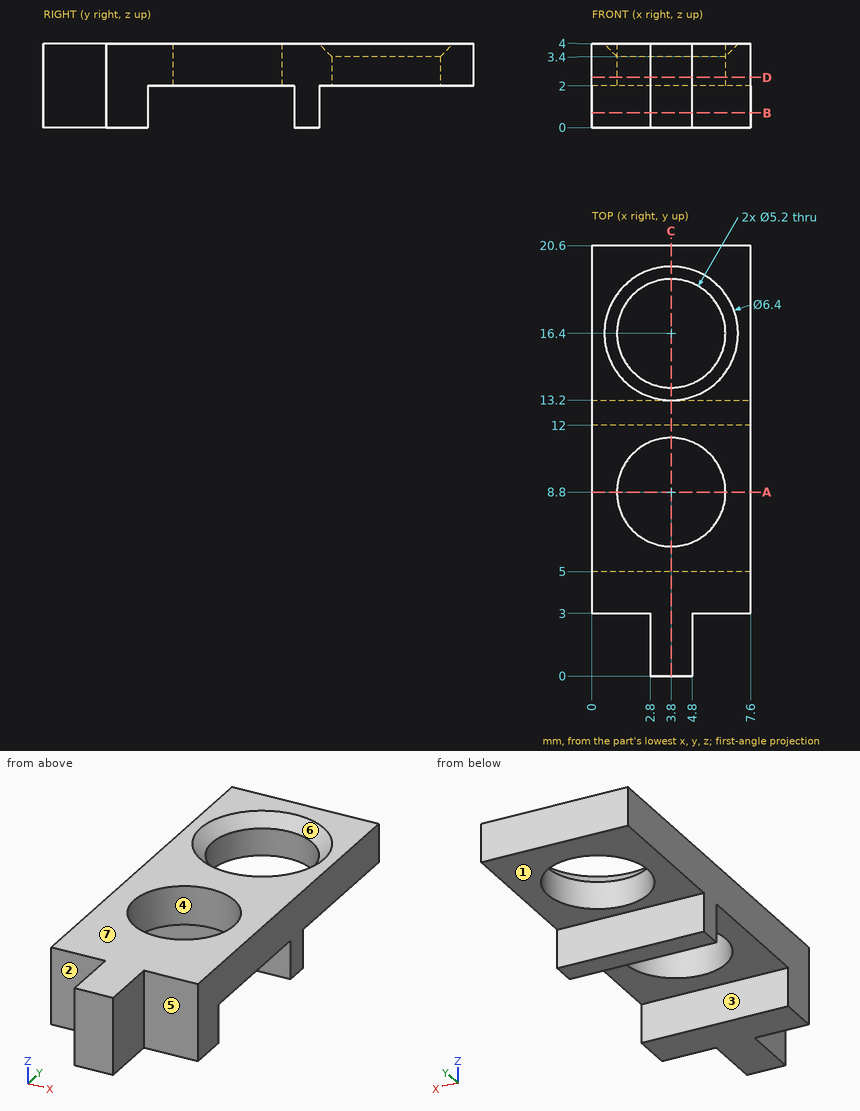
Answer from the drawing. Dimensions are ordinates in mm from the lowest x, y and z of the part. A direction names the side the tool comes from. Give positions to 0.01 mm unless a question says otherwise; leave off trailing zeros. Write each loop counter-clockwise with the first axis right and the second up, starting at its lowest first coordinate (ties: lowest second). Pieces come first, ordered by that corner, then holes. Notation, with made-up numbers: (66.25, -5.75) - (124.25, -5.75) arc R14 cw to (124.25, 16.25) - close; hole circle Ø10 at (82.5, 57.5). An arc over 180 degrees is marked (long way). One line per item, written item: value. Start each with the question number.
1. For the marked faces 1, 2 and 3, determine the directions among +Z, -Z, +X, -X, +Y, -Y from which every point of the face is accessible in a straight line to the end or side of a thin tool.
2. Consider probe 1 along Y at (x, z) = (3.8, 3.1); probe 2 along Y at (x, z) = (6.25, 0.2); probe 3 along Y at (x, z) = (3.5, 0.5). Determine where each line is inside the solid, lowest interval first.
3. Given pin 1 (3.5 mm diameter, centred on x = 3, y = 15, fed in from -Z); pin 2 (1.4 mm diameter, centred on x = 1, z = 1.5, fed in from -Y); pin 3 (0.9 mm diameter, centred on y = 2, z = 1.5, fed in from +X), each flat-ended and moving along its own axis, determine where each tip first touches the part or whether it passes through.
4. Find section A-A (y = 8.8). Write down the section's boundary in (x, z), then the cut area to 3 significant figures.
5. Find section D-D (z = 2.4). Write down the section's boundary in (x, y), then the cut area to 3 significant figures.
6. Find section C-C (x = 3.8). Write down the section's boundary in (y, z), then the cut area to 3 significant figures.
7. Find section B-B (z = 0.7). Write down the section's boundary in (x, y), then the cut area to 3 significant figures.
8. For a pull along Y with two mould halves and no side action, classify the marked faces 4, 5, 6 and 7 as +Y half, -Y half, draft (parallel to the pull), parting line (faces both ways), or undercut.
Geometry results:
1. face 1: -Z, +X, -X, +Y
1. face 2: +Z, -Z, -X, -Y
1. face 3: -Z, +X, -X
2. probe 1: 0 to 6.2, 11.4 to 13.8, 19 to 20.6
2. probe 2: 3 to 5, 12 to 13.2
2. probe 3: 0 to 5, 12 to 13.2
3. pin 1: z = 2
3. pin 2: y = 3
3. pin 3: x = 4.8
4. outline: (0, 2) - (1.2, 2) - (1.2, 4) - (0, 4) - close; (6.4, 2) - (7.6, 2) - (7.6, 4) - (6.4, 4) - close
4. area: 4.80 mm2
5. outline: (0, 3) - (2.8, 3) - (2.8, 0) - (4.8, 0) - (4.8, 3) - (7.6, 3) - (7.6, 20.6) - (0, 20.6) - close; hole circle Ø5.2 at (3.8, 8.8); hole circle Ø5.2 at (3.8, 16.4)
5. area: 97.3 mm2
6. outline: (0, 0) - (5, 0) - (5, 2) - (6.2, 2) - (6.2, 4) - (0, 4) - close; (11.4, 2) - (12, 2) - (12, 0) - (13.2, 0) - (13.2, 2) - (13.8, 2) - (13.8, 3.4) - (13.2, 4) - (11.4, 4) - close; (19, 2) - (20.6, 2) - (20.6, 4) - (19.6, 4) - (19, 3.4) - close
6. area: 32.4 mm2
7. outline: (0, 3) - (2.8, 3) - (2.8, 0) - (4.8, 0) - (4.8, 3) - (7.6, 3) - (7.6, 5) - (0, 5) - close; (0, 12) - (7.6, 12) - (7.6, 13.2) - (0, 13.2) - close
7. area: 30.3 mm2
8. face 4: undercut
8. face 5: -Y half
8. face 6: undercut
8. face 7: draft
